Could you check a few things on this model? Use its own coordinates, in mm. Coordinates: 2 decimals unless noted, no trailing zeros. Write each loop counter-clockwise with the first axis right and the second up, starting at its lowest first coordinate (ties: lowest second). Pieces come first, ordered by that corner, then holes.
Item 1: If I drill on probe 1 along X at (y, z) = (-13, 0.8); probe 2 along Y at (x, z) = (7.5, 0.25); probe 3 along X at (y, z) = (20, 0.7), over which ranges is the centre line in solid material (lowest first)?
Item 2: I want a section at C-C on z = 0.3. State how many separate pieces and enclosed holes the cut face has, then the cut area to 3 significant figures.
Item 3: For P1, Ø0.7, axis at y = 20, z = 1, coming from the +X side, with a flat end and sliding along its axis, tell me the tip position at first contact or that it passes through.
Item 4: I want a section at A-A on x = -21. Please give me the cut outline in (y, z), then the cut area to 3 significant figures.
Item 5: I want a section at B-B on x = 10. Please give me the cut outline in (y, z), then the cut area to 3 significant figures.
from build123d import *

# Parameters (mm, degrees)
CROQUIS1_R              = 1.5621
CROQUIS1_W              = 20.7518
CROQUIS1_H              = 2.4638
CROQUIS1_W_2            = 4.9784
CROQUIS1_H_2            = 46.2788
CROQUIS1_W_3            = 20.828
CROQUIS1_W_4            = 15.6972
CROQUIS1_H_3            = 2.449418676
SALIENTE_EXTRUIR1_DEPTH = 1.55
CROQUIS2_W              = 5
CROQUIS2_H              = 46.2788
CORTAR_EXTRUIR1_DEPTH   = 95.55
CROQUIS3_W              = 0.64
CROQUIS3_H              = 0.64
SALIENTE_EXTRUIR2_DEPTH = 1.55
CROQUIS3_3_W            = 0.64
CROQUIS3_3_H            = 0.64
CROQUIS3_3_H_2          = 0.640713362
SALIENTE_EXTRUIR3_DEPTH = 1.55


with BuildPart() as part:
    # Croquis1 → Saliente-Extruir1 (new body)
    with BuildSketch(Plane.XY):
        Polygon((46.546610497, 27.60316171), (48.310045797, 25.83972641), (48.310045797, 14.90316171), (50.850045797, 12.36316171), (50.850045797, -22.25703829), (47.294045797, -25.81303829), (-49.225954203, -25.81303829), (-50.749954203, -24.28903829), (-50.749954203, -22.00303829), (-50.749954203, -12.85903829), (-50.749954203, 6.39416171), (-50.749954203, 18.33216171), (-50.749954203, 26.07916171), (-49.225954203, 27.60316171), align=None)
        with Locations(Location((-36.627554203, -23.27303829, 0), (0, 0, 180))):
            Circle(CROQUIS1_R, mode=Mode.SUBTRACT)
        with Locations(Location((14.997945797, -18.394545523, 0), (0, 0, 180))):
            Circle(CROQUIS1_R, mode=Mode.SUBTRACT)
        with Locations(Location((45.998645797, -23.27303829, 0), (0, 0, 180))):
            Circle(CROQUIS1_R, mode=Mode.SUBTRACT)
        with Locations(Location((-36.627554203, 25.06316171, 0), (0, 0, 180))):
            Circle(CROQUIS1_R, mode=Mode.SUBTRACT)
        with Locations(Location((38.505645797, 25.06316171, 0), (0, 0, 180))):
            Circle(CROQUIS1_R, mode=Mode.SUBTRACT)
        with Locations((-19.114254203, 25.10126171)):
            Rectangle(CROQUIS1_W, CROQUIS1_H, mode=Mode.SUBTRACT)
        with Locations((3.618745797, 25.10126171)):
            Rectangle(CROQUIS1_W, CROQUIS1_H, mode=Mode.SUBTRACT)
        with Locations((26.351745797, 25.10126171)):
            Rectangle(CROQUIS1_W, CROQUIS1_H, mode=Mode.SUBTRACT)
        with Locations((44.296845797, 3.24456171)):
            Rectangle(CROQUIS1_W_2, CROQUIS1_H_2, mode=Mode.SUBTRACT)
        with Locations((32.181045797, -23.23493829)):
            Rectangle(CROQUIS1_W_3, CROQUIS1_H, mode=Mode.SUBTRACT)
        with Locations((9.448045797, -23.23493829)):
            Rectangle(CROQUIS1_W_3, CROQUIS1_H, mode=Mode.SUBTRACT)
        with Locations((-10.973554203, -23.242128952)):
            Rectangle(CROQUIS1_W_4, CROQUIS1_H_3, mode=Mode.SUBTRACT)
    extrude(amount=SALIENTE_EXTRUIR1_DEPTH)

    # Croquis2 → Cortar-Extruir1 (cut)
    with BuildSketch(Plane(origin=(0, 0, 0), x_dir=(-1, 0, 0), z_dir=(0, 0, -1))):
        with Locations((-44.286045797, 3.24456171)):
            Rectangle(CROQUIS2_W, CROQUIS2_H)
    extrude(amount=-CORTAR_EXTRUIR1_DEPTH, mode=Mode.SUBTRACT)

    # Croquis3 → Saliente-Extruir2 (add)
    with BuildSketch(Plane(origin=(0, 0, 0), x_dir=(-1, 0, 0), z_dir=(0, 0, -1))):
        Polygon((-45.85862689, -7.83483829), (-46.786045797, -7.83483829), (-46.786045797, -19.89483829), (-41.786045797, -19.89483829), (-41.786045797, -7.83483829), (-42.720004997, -7.83483829), (-42.720004997, -8.15483829), (-43.360004997, -8.15483829), (-43.360004997, -7.83483829), (-45.218685961, -7.83483829), (-45.218685961, -8.15483829), (-45.85862689, -8.15483829), align=None)
        with Locations((-45.538685961, -17.99483829)):
            Rectangle(CROQUIS3_W, CROQUIS3_H, mode=Mode.SUBTRACT)
        with Locations((-43.040004997, -17.99483829)):
            Rectangle(CROQUIS3_W, CROQUIS3_H, mode=Mode.SUBTRACT)
        with Locations((-45.538685961, -15.45483829)):
            Rectangle(CROQUIS3_W, CROQUIS3_H, mode=Mode.SUBTRACT)
        with Locations((-45.538685961, -12.91483829)):
            Rectangle(CROQUIS3_W, CROQUIS3_H, mode=Mode.SUBTRACT)
        with Locations((-43.040004997, -15.45483829)):
            Rectangle(CROQUIS3_W, CROQUIS3_H, mode=Mode.SUBTRACT)
        with Locations((-43.040004997, -12.91483829)):
            Rectangle(CROQUIS3_W, CROQUIS3_H, mode=Mode.SUBTRACT)
        with Locations((-45.538685961, -10.37483829)):
            Rectangle(CROQUIS3_W, CROQUIS3_H, mode=Mode.SUBTRACT)
        with Locations((-43.040004997, -10.37483829)):
            Rectangle(CROQUIS3_W, CROQUIS3_H, mode=Mode.SUBTRACT)
    extrude(amount=-SALIENTE_EXTRUIR2_DEPTH)

    # Croquis3<3> → Saliente-Extruir3 (add)
    with BuildSketch(Plane(origin=(0, 0, 0), x_dir=(-1, 0, 0), z_dir=(0, 0, -1))):
        Polygon((-46.786045797, 26.38396171), (-46.786045797, -7.83483829), (-45.85862689, -7.83483829), (-45.85862689, -7.51483829), (-45.218685961, -7.51483829), (-45.218685961, -7.83483829), (-43.360004997, -7.83483829), (-43.360004997, -7.51483829), (-42.720004997, -7.51483829), (-42.720004997, -7.83483829), (-41.786045797, -7.83483829), (-41.786045797, 26.38396171), align=None)
        with Locations((-45.538685961, -5.29483829)):
            Rectangle(CROQUIS3_3_W, CROQUIS3_3_H, mode=Mode.SUBTRACT)
        with Locations((-45.538685961, -2.75483829)):
            Rectangle(CROQUIS3_3_W, CROQUIS3_3_H, mode=Mode.SUBTRACT)
        with Locations((-43.040004997, -5.29483829)):
            Rectangle(CROQUIS3_3_W, CROQUIS3_3_H, mode=Mode.SUBTRACT)
        with Locations((-43.040004997, -2.75483829)):
            Rectangle(CROQUIS3_3_W, CROQUIS3_3_H, mode=Mode.SUBTRACT)
        with Locations((-45.538685961, -0.21483829)):
            Rectangle(CROQUIS3_3_W, CROQUIS3_3_H, mode=Mode.SUBTRACT)
        with Locations((-43.040004997, -0.21483829)):
            Rectangle(CROQUIS3_3_W, CROQUIS3_3_H, mode=Mode.SUBTRACT)
        with Locations((-45.538685961, 2.32516171)):
            Rectangle(CROQUIS3_3_W, CROQUIS3_3_H, mode=Mode.SUBTRACT)
        with Locations((-43.040004997, 2.32516171)):
            Rectangle(CROQUIS3_3_W, CROQUIS3_3_H, mode=Mode.SUBTRACT)
        with Locations((-45.538685961, 4.86516171)):
            Rectangle(CROQUIS3_3_W, CROQUIS3_3_H, mode=Mode.SUBTRACT)
        with Locations((-45.538685961, 7.40516171)):
            Rectangle(CROQUIS3_3_W, CROQUIS3_3_H, mode=Mode.SUBTRACT)
        with Locations((-43.040004997, 4.86516171)):
            Rectangle(CROQUIS3_3_W, CROQUIS3_3_H, mode=Mode.SUBTRACT)
        with Locations((-43.040004997, 7.40516171)):
            Rectangle(CROQUIS3_3_W, CROQUIS3_3_H, mode=Mode.SUBTRACT)
        with Locations((-45.538685961, 9.94516171)):
            Rectangle(CROQUIS3_3_W, CROQUIS3_3_H, mode=Mode.SUBTRACT)
        with Locations((-43.040004997, 9.94516171)):
            Rectangle(CROQUIS3_3_W, CROQUIS3_3_H, mode=Mode.SUBTRACT)
        with Locations((-45.538685961, 12.48516171)):
            Rectangle(CROQUIS3_3_W, CROQUIS3_3_H, mode=Mode.SUBTRACT)
        with Locations((-43.040004997, 12.48516171)):
            Rectangle(CROQUIS3_3_W, CROQUIS3_3_H, mode=Mode.SUBTRACT)
        with Locations((-45.538685961, 15.02516171)):
            Rectangle(CROQUIS3_3_W, CROQUIS3_3_H, mode=Mode.SUBTRACT)
        with Locations((-45.538685961, 17.56516171)):
            Rectangle(CROQUIS3_3_W, CROQUIS3_3_H, mode=Mode.SUBTRACT)
        with Locations((-43.040004997, 15.02516171)):
            Rectangle(CROQUIS3_3_W, CROQUIS3_3_H, mode=Mode.SUBTRACT)
        with Locations((-43.040004997, 17.56516171)):
            Rectangle(CROQUIS3_3_W, CROQUIS3_3_H, mode=Mode.SUBTRACT)
        with Locations((-45.538685961, 20.10516171)):
            Rectangle(CROQUIS3_3_W, CROQUIS3_3_H, mode=Mode.SUBTRACT)
        with Locations((-43.040004997, 20.18636171)):
            Rectangle(CROQUIS3_3_W, CROQUIS3_3_H_2, mode=Mode.SUBTRACT)
        with Locations((-45.538685961, 22.64516171)):
            Rectangle(CROQUIS3_3_W, CROQUIS3_3_H, mode=Mode.SUBTRACT)
        with Locations((-43.036045797, 22.64516171)):
            Rectangle(CROQUIS3_3_W, CROQUIS3_3_H, mode=Mode.SUBTRACT)
        with Locations((-45.538685961, 25.18516171)):
            Rectangle(CROQUIS3_3_W, CROQUIS3_3_H, mode=Mode.SUBTRACT)
        with Locations((-43.040004997, 25.10396171)):
            Rectangle(CROQUIS3_3_W, CROQUIS3_3_H_2, mode=Mode.SUBTRACT)
    extrude(amount=-SALIENTE_EXTRUIR3_DEPTH)


solid = part.part
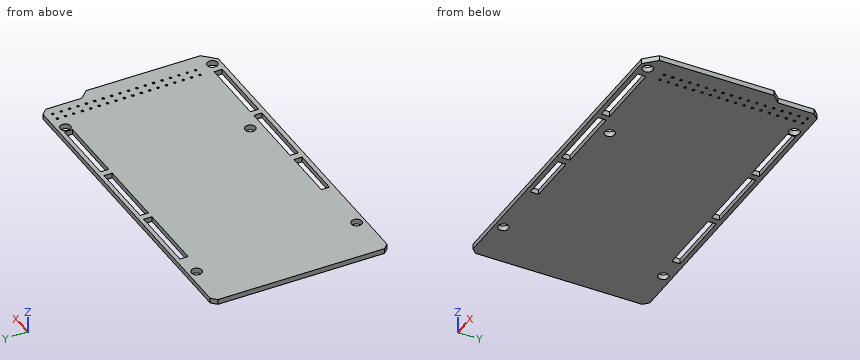
Response values:
1. probe 1: x = -50.75 to 42.72, 43.36 to 45.22, 45.86 to 50.85
1. probe 2: y = -25.81 to -24.47, -22 to 23.87, 26.33 to 27.6
1. probe 3: x = -50.75 to 42.72, 43.36 to 45.22, 45.86 to 48.31
2. separate pieces: 1
2. enclosed holes: 47
2. area: 5,030 mm2
3. P1: stops at x = 48.31
4. outline: (-25.81, 0) - (23.87, 0) - (23.87, 1.55) - (-25.81, 1.55) - close; (26.33, 0) - (27.6, 0) - (27.6, 1.55) - (26.33, 1.55) - close
4. area: 79.0 mm2
5. outline: (-25.81, 0) - (-24.47, 0) - (-24.47, 1.55) - (-25.81, 1.55) - close; (-22, 0) - (23.87, 0) - (23.87, 1.55) - (-22, 1.55) - close; (26.33, 0) - (27.6, 0) - (27.6, 1.55) - (26.33, 1.55) - close
5. area: 75.2 mm2
